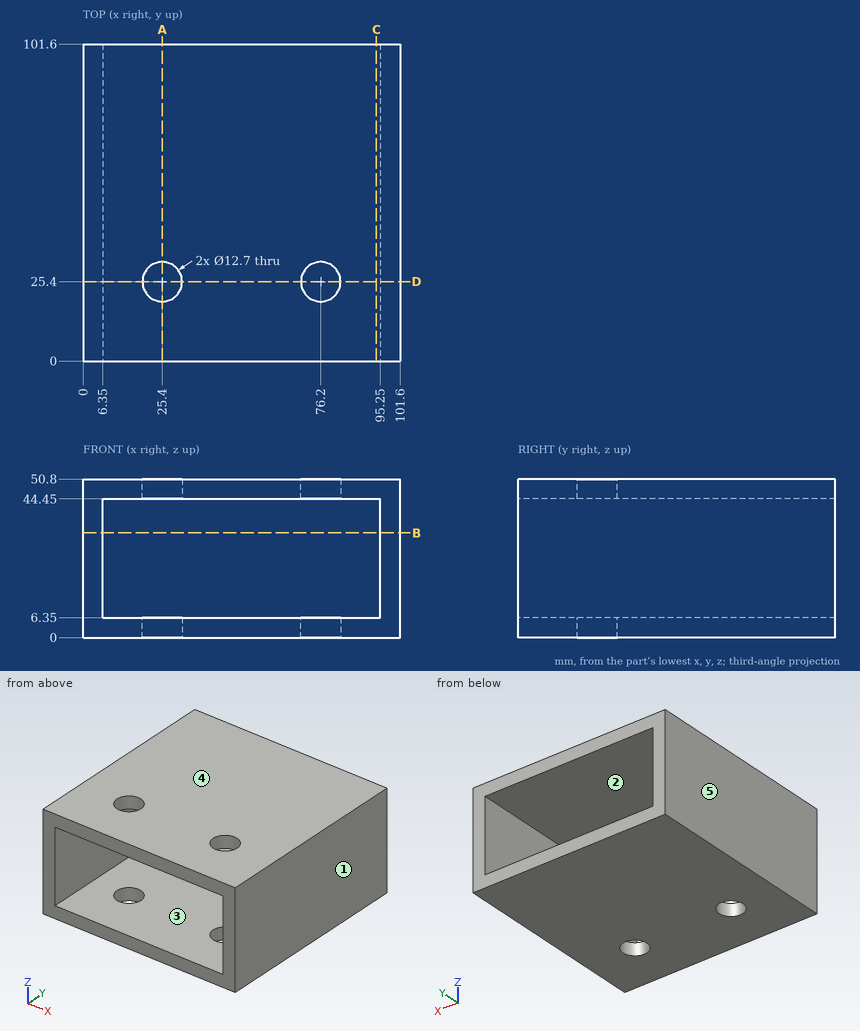
Verification items for this drawing (mm, ordinates from the low corner). A direction names the side the tool comes from. Coordinates: 2 decimals unless noted, no trailing zeros. Order: outer loops, then holes, each group sorted by start corner. A loop starts at its lowest first (then second) coordinate and runs counter-clockwise, first axis right, second up. Notation, with made-up numbers: M 4.5,-16 L 61.5,-16 A12 cw 61.5,7 Z; hole C -29.5,47.25 d10. An arc over 180 degrees is marked long. Write each question's results on one line, items separated by ' | '.
1) Access from +Z, -Z, +X, -X, +Y, -Y to the whole of each face (thin tool, end or side, straight path). Record for the marked faces 1 and 2.
Solved:
face 1: +Z, -Z, +X, +Y, -Y | face 2: +Y, -Y
2) Gauge pin test, flat end, axial feed: pin 1 Ø10 at (x, y) = (76.2, 25.4) entering from -Z. Record the tip position at first contact, or that the pin passes through.
Solved:
pin 1: passes through
3) Section check C-C on x = 94. Record the cut outline in (y, z), plus the area to 3 significant figures.
Solved:
outline: M 0,0 L 101.6,0 L 101.6,6.35 L 0,6.35 Z; M 0,44.45 L 101.6,44.45 L 101.6,50.8 L 0,50.8 Z | area: 1,290 mm²
4) Section check B-B on z = 33.5. Record the cut outline in (x, y), plus the area to 3 significant figures.
Solved:
outline: M 0,0 L 6.35,0 L 6.35,101.6 L 0,101.6 Z; M 95.25,0 L 101.6,0 L 101.6,101.6 L 95.25,101.6 Z | area: 1,290 mm²
5) Scan lines: line 1 along X through (y, z) = (25, 1); line 2 along Z through (x, y) = (27, 36); line 3 along Y through (x, z) = (76, 46). Record each from-to range of solid material in increasing order. Write a range as [from, to].
Solved:
line 1: x = [0, 19.06], [31.74, 69.86], [82.54, 101.6] | line 2: z = [0, 6.35], [44.45, 50.8] | line 3: y = [0, 19.05], [31.75, 101.6]
6) Release check for a two-part mould opening along X. For the marked faces 3, 4 and 5 record: pulls with the +X half, pulls with the -X half, needs draft (parallel to the pull), parting line crosses it, or undercut.
Solved:
face 3: undercut | face 4: needs draft | face 5: pulls with the -X half
7) Section check A-A on x = 25.4. Record the cut outline in (y, z), plus the area to 3 significant figures.
Solved:
outline: M 0,0 L 19.05,0 L 19.05,6.35 L 0,6.35 Z; M 0,44.45 L 19.05,44.45 L 19.05,50.8 L 0,50.8 Z; M 31.75,0 L 101.6,0 L 101.6,6.35 L 31.75,6.35 Z; M 31.75,44.45 L 101.6,44.45 L 101.6,50.8 L 31.75,50.8 Z | area: 1,130 mm²
8) Section check D-D on y = 25.4. Record the cut outline in (x, z).
Solved:
outline: M 0,0 L 19.05,0 L 19.05,6.35 L 6.35,6.35 L 6.35,44.45 L 19.05,44.45 L 19.05,50.8 L 0,50.8 Z; M 31.75,0 L 69.85,0 L 69.85,6.35 L 31.75,6.35 Z; M 31.75,44.45 L 69.85,44.45 L 69.85,50.8 L 31.75,50.8 Z; M 82.55,0 L 101.6,0 L 101.6,50.8 L 82.55,50.8 L 82.55,44.45 L 95.25,44.45 L 95.25,6.35 L 82.55,6.35 Z
